Source: three-view drawing plus pictorial views. Frame: mm from the lowest corner of the part. A direction names the side the tool comes from. Give positions to 0.01 mm unless a question says otherwise; leave off trailing zeros. Loops run counter-clockwise (first coordinate to the right, second up) from the corner with the lowest first, then second, coordinate; pieces in that order, holes last. Notation, with made-up numbers: M 32.25,11 L 73.25,11 A12 ccw 73.25,32 Z; hole C 70.25,40.25 d3. An arc over 180 degrees is marked long. Answer as a JSON object with one key per item and string values. Group by question number.
1) Section query D-D on x = 93. Return loops of the section in (y, z).
2) Ray query, L1, parallel to X at y = 38.5, z = 26; L2, parallel to Y at x = 100.5, z = 13.5; L3, parallel to Y at x = 59, z = 24.5. Return the intervals inside material, ascending.
3) Section query C-C on y = 30.5. Return loops of the section in (x, z), plus the area to 3 significant figures.
4) Section query B-B on x = 41. Return loops of the section in (y, z).
5) Access query for the marked faces 1 and 2. Directions: +Z, -Z, +X, -X, +Y, -Y. A direction counts if a zero-diameter tool reaches every point of the face in a straight line with its end or side. Return the directions, or none.
6) First-contact query: P1, Ø4, axis at y = 13, z = 18, coming from the -X side; P2, Ø3, axis at x = 124, z = 31, coming from the -Y side; P3, Ø2, axis at x = 39.5, z = 18.5, coming from the -Y side; P4, Ø15, axis at y = 14.5, z = 36.5, coming from the +X side. Flat tips, straight axial feed; report the tip coordinate or a pass-through.
7) Section query A-A on z = 20. Return loops of the section in (x, y).
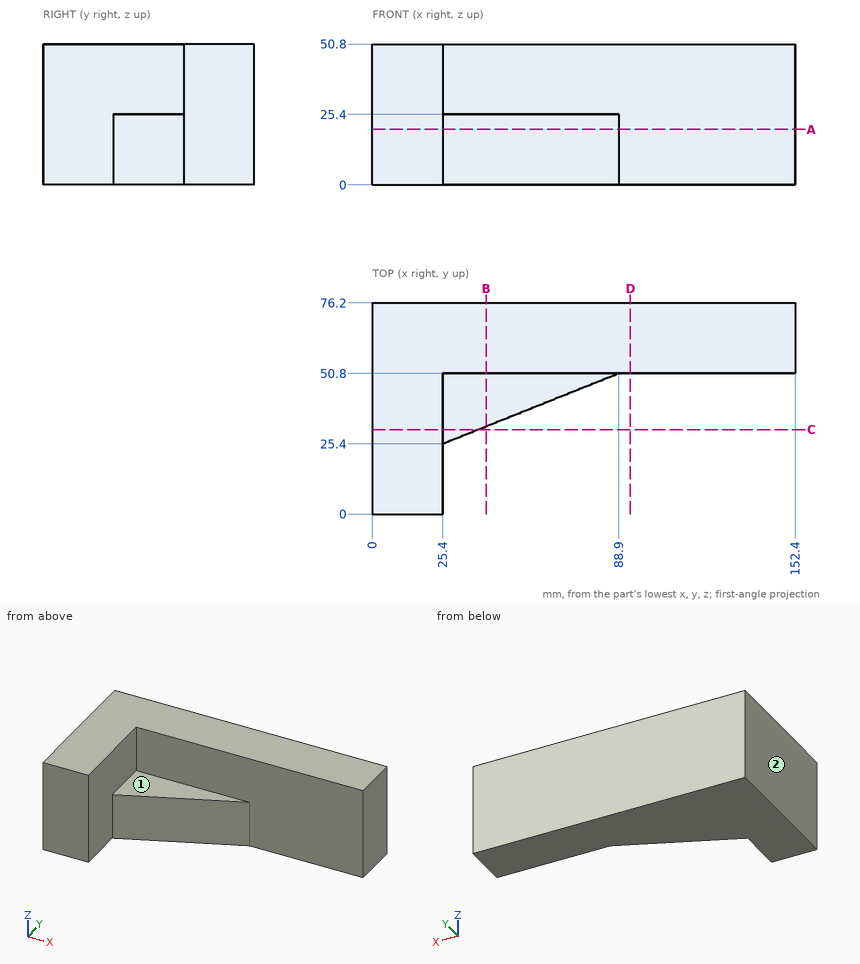
Output:
{
 "1": {"outline": "M 50.8,0 L 76.2,0 L 76.2,50.8 L 50.8,50.8 Z"},
 "2": {"L1": "x = 0 to 25.4", "L2": "y = 50.8 to 76.2", "L3": "y = 38.84 to 76.2"},
 "3": {"outline": "M 0,0 L 38.15,0 L 38.15,25.4 L 25.4,25.4 L 25.4,50.8 L 0,50.8 Z", "area": "1,610 mm^2"},
 "4": {"outline": "M 31.64,0 L 76.2,0 L 76.2,50.8 L 50.8,50.8 L 50.8,25.4 L 31.64,25.4 Z"},
 "5": {"face 1": "+Z, +X, -Y", "face 2": "+Z, -Z, -X, +Y, -Y"},
 "6": {"P1": "stops at x = 0", "P2": "stops at y = 50.8", "P3": "stops at y = 30.64", "P4": "stops at x = 25.4"},
 "7": {"outline": "M 0,0 L 25.4,0 L 25.4,25.4 L 88.9,50.8 L 152.4,50.8 L 152.4,76.2 L 0,76.2 Z"}
}
